Autodesk Inventor part; units mm, degrees
ref_plane "YZ Plane" through (0, 0, 0) normal (1, 0, 0) x (0, 1, 0)
ref_plane "XZ Plane" through (0, 0, 0) normal (0, 1, 0) x (-1, 0, 0)
ref_plane "XY Plane" through (0, 0, 0) normal (0, 0, 1) x (1, 0, 0)
sketch "Sketch1" plane through (0, 0, 0) normal (0, 0, 1) x (1, 0, 0)
  line L0 (-6.35, -6.35) -> (6.35, -6.35)
  line L1 (6.35, -6.35) -> (6.35, 6.35)
  line L2 (6.35, 6.35) -> (-6.35, 6.35)
  line L3 (-6.35, 6.35) -> (-6.35, -6.35)
  line L4 (-6.35, -6.35) -> (6.35, 6.35) construction
  line L5 (6.35, -6.35) -> (-6.35, 6.35) construction
  line L6 (4.572, 4.572) -> (-4.572, 4.572)
  line L7 (-4.572, 4.572) -> (-4.572, -4.572)
  line L8 (-4.572, -4.572) -> (4.572, -4.572)
  line L9 (4.572, -4.572) -> (4.572, 4.572)
  line L10 (4.572, 4.572) -> (-4.572, -4.572) construction
  line L11 (-4.572, 4.572) -> (4.572, -4.572) construction
  point P0 (0, 0)
  dimension "d0" = 12.7
  dimension "d1" = 12.7
  dimension "d2" = 10.922
  dimension "d3" = 10.922
extrude "Extrusion1" add sketch "Sketch1" along normal blind 152.4
sketch "Sketch2" plane through (6.35, -6.35, 0) normal (1, 0, 0) x (0, 0, -1)
  line L0 (0, 0) -> (0, 12.7)
  line L1 (-152.4, 0) -> (-152.4, 12.7)
  circle A0 centre (-146.05, 6.35) radius 2.1336
  circle A1 centre (-6.35, 6.35) radius 2.1336
  point P0 (0, 6.35)
  dimension "d6" = 4.2672
  dimension "d7" = 6.35
  dimension "d8" = 4.2672
  dimension "d9" = 6.35
extrude "Extrusion2" cut sketch "Sketch2" against normal blind 12.7
properties part number "ShortBox" material "Aluminum 6061"
Work out the finished part from the listing and answer in its coordinate system (mm). A direction names the side the tool comes from. Round coordinates to 2 decimals unless told otherwise and drop trailing zeros. Loops run counter-clockwise (first coordinate to the right, second up) from the corner with the lowest first, then second, coordinate; pieces in that order, holes last. Notation, with made-up numbers: (49.5, 43.25) - (99.5, 43.25) arc R21 ccw to (99.5, 81.25) - close; hole circle Ø1 at (74.5, 61). An arc over 180 degrees is marked (long way). Use one line per item in the form item = value. Start each with the question number.
(1) Determine the mould class of faces 1 (the face through (0, 4.572, 75)), 2 (the face through (5.47, -1.3, 8.04)), 3 (the face through (6.35, 0, 75)), 4 (the face through (-6.35, 0, 75)) for opening direction X: +X half, -X half, draft (parallel to the pull), parting line (faces both ways), or undercut.
(2) Find section C-C on y = 0. Determine the outline of the cut face in (x, z), and give its area (3 significant figures).
(3) Find section B-B on z = 22.5. Determine the outline of the cut face in (x, y).
(4) Consider line 1 (X direction, y = 2.5, z = 60.5); line 2 (Y direction, x = -5.05, z = 146.05). Determine where each line is inside the solid, lowest interval first.
(5) Which of the six approach directions +Z, -Z, +X, -X, +Y, -Y give full straight-line access (tool end or side, diameter ignored) to faces 5 (the face through (6, 0, 0)), 6 (the face through (4.572, 0, 75))?
(6) Find section D-D on z = 146.05. Determine the outline of the cut face in (x, y).
(7) Find section A-A on x = -1. Determine the outline of the cut face in (y, z), and give its area (3 significant figures).
(8) A flat-ended cylindrical pin translates along its axis: P1, Ø3.5, axis at y = 0, z = 6.35, coming from the -X side. Find the tip coordinate at first contact, or state that the pin passes through.
Answer list:
q1.face_1 = undercut
q1.face_2 = draft
q1.face_3 = +X half
q1.face_4 = -X half
q2.outline = (-6.35, 0) - (-4.57, 0) - (-4.57, 4.22) - (-6.35, 4.22) - close; (-6.35, 8.48) - (-4.57, 8.48) - (-4.57, 143.92) - (-6.35, 143.92) - close; (-6.35, 148.18) - (-4.57, 148.18) - (-4.57, 152.4) - (-6.35, 152.4) - close; (4.57, 0) - (6.35, 0) - (6.35, 4.22) - (4.57, 4.22) - close; (4.57, 8.48) - (6.35, 8.48) - (6.35, 143.92) - (4.57, 143.92) - close; (4.57, 148.18) - (6.35, 148.18) - (6.35, 152.4) - (4.57, 152.4) - close
q2.area = 512 mm^2
q3.outline = (-6.35, -6.35) - (6.35, -6.35) - (6.35, 6.35) - (-6.35, 6.35) - close; hole (-4.57, -4.57) - (4.57, -4.57) - (4.57, 4.57) - (-4.57, 4.57) - close
q4.line_1 = -6.35 to -4.57, 4.57 to 6.35
q4.line_2 = -6.35 to -2.13, 2.13 to 6.35
q5.face_5 = -Z, +X, -X, +Y, -Y
q5.face_6 = +Z, -Z
q6.outline = (-6.35, -6.35) - (6.35, -6.35) - (6.35, -2.13) - (4.57, -2.13) - (4.57, -4.57) - (-4.57, -4.57) - (-4.57, -2.13) - (-6.35, -2.13) - close; (-6.35, 2.13) - (-4.57, 2.13) - (-4.57, 4.57) - (4.57, 4.57) - (4.57, 2.13) - (6.35, 2.13) - (6.35, 6.35) - (-6.35, 6.35) - close
q7.outline = (-6.35, 0) - (-4.57, 0) - (-4.57, 152.4) - (-6.35, 152.4) - close; (4.57, 0) - (6.35, 0) - (6.35, 152.4) - (4.57, 152.4) - close
q7.area = 542 mm^2
q8.P1 = through
